from build123d import *

# Parameters (mm, degrees)
F1_R     = 4.5
F2_DEPTH = 9
F3_R     = 1.5
F4_DEPTH = 12
F0_R     = 0.5


with BuildPart() as f2:
    # F1 (on Top) → F2 (new body)
    with BuildSketch(Plane.XY):
        Circle(F1_R)
    extrude(amount=F2_DEPTH)

    # F3 (on face) → F4 (join)
    with BuildSketch(Plane(origin=(0, 0, 0), x_dir=(1, 0, 0), z_dir=(0, 0, -1))):
        Circle(F3_R)
    extrude(amount=F4_DEPTH)

    # F0
    f0_edges = [f2.edges().sort_by_distance(p)[0] for p in [
        (-4.5, 0, 9),
        (-1.5, 0, -12),
    ]]
    fillet(f0_edges, radius=F0_R)


solid = f2.part
Read the model definition and answer for the solid it produces. Units are mm, in the model's axes. A direction names the side the tool comes from. Coordinates: 2 decimals unless noted, no trailing zeros. Order: outer loops, then holes, each group sorted by start corner. A loop starts at its lowest first (then second) coordinate and runs counter-clockwise, first axis right, second up. Notation, with made-up numbers: M -1.5,-21.75 L 53.5,-21.75 A31 ccw 53.5,2.25 Z; hole C -25.5,-34 d3. An arc over 180 degrees is marked long. Put each result on its own line as item: value. Start each with the question number.
Item 1: Given pin 1 Ø4 at (y, z) = (-2, 6.5) entering from -X; pin 2 Ø2 at (y, z) = (0, -1.5) entering from -X; pin 3 Ø1.5 at (x, z) = (-3, -5) entering from -Y, each flat-ended and moving along its own axis, determine where each tip first touches the part or whether it passes through.
Item 2: Section A-A, the plane x = 0 is taken. Determine the outline of the cut face in (y, z).
Item 3: Consider probe 1 along Z at (x, y) = (1.75, -3.5); probe 2 along X at (y, z) = (0, -4.5); probe 3 along Z at (x, y) = (-3.5, 2.75). Determine where each line is inside the solid, lowest interval first. Write a range as [from, to].
Item 4: For faces 1 (the face through (0, 0, -12)), 2 (the face through (-1.5, -0.07, -5.67)), determine the directions among +Z, -Z, +X, -X, +Y, -Y from which every point of the face is accessible in a straight line to the end or side of a thin tool.
Item 5: Section C-C, the plane z = 5.5 is taken. Determine the outline of the cut face in (x, y), plus the area to 3 significant figures.
Item 6: Section D-D, the plane z = -7.5 is taken. Determine the outline of the cut face in (x, y).
Computed:
1. pin 1: stops at x = -4.5
1. pin 2: stops at x = -1.5
1. pin 3: passes through
2. outline: M -4.5,0 L -1.5,0 L -1.5,-11.5 A0.5 ccw -1,-12 L 1,-12 A0.5 ccw 1.5,-11.5 L 1.5,0 L 4.5,0 L 4.5,8.5 A0.5 ccw 4,9 L -4,9 A0.5 ccw -4.5,8.5 Z
3. probe 1: z = [0, 9]
3. probe 2: x = [-1.5, 1.5]
3. probe 3: z = [0, 8.72]
4. face 1: -Z, +X, -X, +Y, -Y
4. face 2: -Z
5. outline: C 0,0 d9
5. area: 63.6 mm2
6. outline: C 0,0 d3
